Autodesk Inventor part; units mm, degrees
ref_plane "YZ Plane" through (0, 0, 0) normal (1, 0, 0) x (0, 1, 0)
ref_plane "XZ Plane" through (0, 0, 0) normal (0, 1, 0) x (-1, 0, 0)
ref_plane "XY Plane" through (0, 0, 0) normal (0, 0, 1) x (1, 0, 0)
sketch "スケッチ1" plane through (0, 0, 0) normal (0, 1, 0) x (-1, 0, 0)
  circle A0 centre (0, 0) radius 2
  dimension "d0" = 4
extrude "押し出し1" add sketch "スケッチ1" against normal blind 8
sketch "スケッチ2" plane through (0, 0, 0) normal (0, 1, 0) x (1, 0, 0)
  circle A0 centre (0, 0) radius 2
  circle A1 centre (0, 0) radius 3.5
  dimension "d3" = 7
extrude "押し出し2" add sketch "スケッチ2" along normal blind 4 contours A0 | A1
sketch "スケッチ3" plane through (0, 4, 0) normal (0, 1, 0) x (1, 0, 0)
  circle A0 centre (0, 0) radius 1.7 construction
  line L0 (0, 1.7) -> (-1.4722, 0.85)
  line L1 (-1.4722, 0.85) -> (-1.4722, -0.85)
  line L2 (-1.4722, -0.85) -> (0, -1.7)
  line L3 (0, -1.7) -> (1.4722, -0.85)
  line L4 (1.4722, -0.85) -> (1.4722, 0.85)
  line L5 (1.4722, 0.85) -> (0, 1.7)
  dimension "d6" = 3.4
  dimension "d9" = 360
extrude "押し出し3" cut sketch "スケッチ3" against normal blind 2.3
chamfer "面取り1" distance 0.2 angle 45 1 edges at (-3.5, 4, 0)
thread "ねじ1"
sketch "スケッチ4" plane through (0, 1.7, 0) normal (0, 1, 0) x (1, 0, 0)
  circle A0 centre (0, 0) radius 0.5
  dimension "d18" = 1
extrude "押し出し4" cut sketch "スケッチ4" against normal through all
properties part number "M4×8-VentedHexSocket" material "ステンレス鋼"
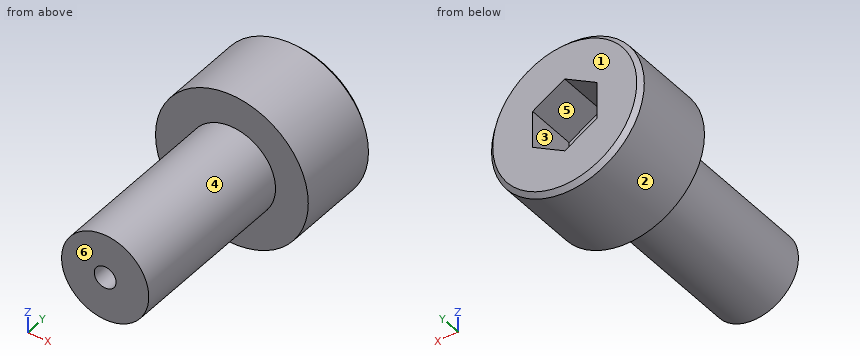
Here's how the part is built. I have some questions about the finished solid (model axes, mm). Face numbers are marked on the shaded views. A direction names the side the tool comes from. Coordinates: 2 decimals unless noted, no trailing zeros. Order: outer loops, then holes, each group sorted by start corner. A loop starts at its lowest first (then second) coordinate and runs counter-clockwise, first axis right, second up. Notation, with made-up numbers: M 72.5,-37 L 111.5,-37 A17 ccw 111.5,-29 Z; hole C 55,71 d6. An arc over 180 degrees is marked long. Answer as a JSON object with one key per item and string values. Group by question number.
(1) Suppose I cut it at D-D, the plane y = -5. Please give me the cut outline in (x, z), then the cut area to 3 significant figures.
(2) Suppose I cut it at C-C, the plane y = 0.75. Please give me the cut outline in (x, z).
(3) Suppose I cut it at A-A, the plane z = 0. Please give me the cut outline in (x, y), then the cut area to 3 significant figures.
(4) Which directions (+Z, -Z, +X, -X, +Y, -Y) give clear straight access to the entire face, cutting with the end or side of a thin tool? Please do the marked faces 4, 5 and 6.
(5) I need wall thicknesses on probe 1 along Z at (x, y) = (0, -3.25); probe 2 along Y at (x, z) = (0.5, 2); probe 3 along Y at (x, z) = (-0.5, -0.25). Which ranges of each line are inside material? Lowest first, please.
(6) For pin 1 (2 mm diameter, centred on x = 0, y = -2.5, fed in from -Z); pin 2 (1.5 mm diameter, centred on x = -0.5, z = -0.5, fed in from +Y); pin 3 (2 mm diameter, centred on x = 2, z = 2.5, fed in from -Y), each with a flat end and sliding along its axis, tell me the tip position at first contact or that it passes through.
(7) If we mould it in two halves opening along X, with no side actions, what happens to the marked faces 1, 2 and 3? For each: released by +X, released by -X, zero draft, split by the parting line, or undercut.
(8) Suppose I cut it at B-B, the plane y = 2.75. Please give me the cut outline in (x, z), then the cut area to 3 significant figures.
Values found:
{
 "1": {"outline": "C 0,0 d4; hole C 0,0 d1", "area": "11.8 mm^2"},
 "2": {"outline": "C 0,0 d7; hole C 0,0 d1"},
 "3": {"outline": "M -3.5,0 L -2,0 L -2,-8 L -0.5,-8 L -0.5,1.7 L -1.47,1.7 L -1.47,4 L -3.3,4 L -3.5,3.8 Z; M 0.5,-8 L 2,-8 L 2,0 L 3.5,0 L 3.5,3.8 L 3.3,4 L 1.47,4 L 1.47,1.7 L 0.5,1.7 Z", "area": "43.5 mm^2"},
 "4": {"face 4": "-Y", "face 5": "+Y", "face 6": "+Z, -Z, +X, -X, -Y"},
 "5": {"probe 1": "z = -2 to -0.5, 0.5 to 2", "probe 2": "y = 0 to 4", "probe 3": "y = -8 to 1.7"},
 "6": {"pin 1": "stops at z = -2", "pin 2": "stops at y = 1.7", "pin 3": "stops at y = 0"},
 "7": {"face 1": "zero draft", "face 2": "split by the parting line", "face 3": "undercut"},
 "8": {"outline": "C 0,0 d7; hole M -1.47,-0.85 L 0,-1.7 L 1.47,-0.85 L 1.47,0.85 L 0,1.7 L -1.47,0.85 Z", "area": "31.0 mm^2"}
}
